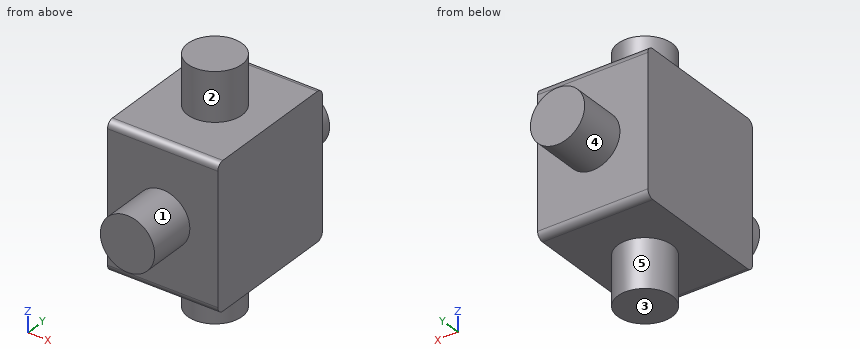
from build123d import *

# Parameters (mm, degrees)
SZKIC1_W                    = 13.2
SZKIC1_H                    = 13.2
DODANIE_WYCI_GNI_CIE1_DEPTH = 10.12
SZKIC2_W                    = 2.49
SZKIC2_H                    = 4.45
SZKIC3_W                    = 2.49
SZKIC3_H                    = 4.45
SZKIC4_W                    = 2.49
SZKIC4_H                    = 4.45
SZKIC5_W                    = 2.49
SZKIC5_H                    = 4.45
ZAOKR_GLENIE1_R             = 0.628571429


with BuildPart() as part:
    # Szkic1 → Dodanie-wyciągnięcie1 (new body)
    with BuildSketch(Plane(origin=(5.06, 0, 0), x_dir=(0, 0, -1), z_dir=(1, 0, 0))):
        Rectangle(SZKIC1_W, SZKIC1_H)
    extrude(amount=-DODANIE_WYCI_GNI_CIE1_DEPTH)

    # Szkic2 → Obrót1 (revolve)
    with BuildSketch(Plane(origin=(0, 0, 0), x_dir=(-1, 0, 0), z_dir=(0, 0, -1))):
        with Locations((-1.245, 8.825)):
            Rectangle(SZKIC2_W, SZKIC2_H)
    revolve(axis=Axis((0, 6.6, 0), (0, 1, 0)))

    # Szkic3 → Obrót2 (revolve)
    with BuildSketch(Plane.XZ):
        with Locations((1.245, -8.825)):
            Rectangle(SZKIC3_W, SZKIC3_H)
    revolve(axis=Axis((0, 0, -6.6), (0, 0, -1)))

    # Szkic4 → Obrót3 (revolve)
    with BuildSketch(Plane(origin=(0, 0, 0), x_dir=(-1, 0, 0), z_dir=(0, 0, -1))):
        with Locations((-1.245, -8.825)):
            Rectangle(SZKIC4_W, SZKIC4_H)
    revolve(axis=Axis((0, -11.05, 0), (0, 1, 0)))

    # Szkic5 → Obrót4 (revolve)
    with BuildSketch(Plane.XZ):
        with Locations((1.245, 8.825)):
            Rectangle(SZKIC5_W, SZKIC5_H)
    revolve(axis=Axis((0, 0, 11.05), (0, 0, -1)))

    # Zaokrąglenie1
    zaokr_glenie1_edges = [part.edges().sort_by_distance(p)[0] for p in [
        (0, 6.6, -6.6),
        (0, -6.6, -6.6),
        (0, -6.6, 6.6),
        (0, 6.6, 6.6),
    ]]
    fillet(zaokr_glenie1_edges, radius=ZAOKR_GLENIE1_R)


solid = part.part
Check sheet for the modelled part. Datum: model origin and axes. Units: mm. Face numbers are marked on the shaded views. A direction names the side the tool comes from. Round coordinates to 2 decimals unless told otherwise and drop trailing zeros. Order: outer loops, then holes, each group sorted by start corner. A loop starts at its lowest first (then second) coordinate and runs counter-clockwise, first axis right, second up. Notation, with made-up numbers: M 44.25,33 L 85.25,33 A21 cw 85.25,48 Z; hole C 29.5,-29.75 d5. An arc over 180 degrees is marked long. One line per item, written item: value. Start each with the question number.
1. Section check A-A on x = 0. Enter the section's corners in (y, z), and give its area (3 significant figures).
2. Gauge pin test, flat ends, axial feed: P1, Ø1, axis at x = -2.5, y = 2.5, coming from the -Z side; P2, Ø2, axis at x = 2, z = -8.5, coming from the +Y side. Record the tip position at first contact, or that the pin passes through.
3. Section check D-D on x = -1.25. Enter the section's corners in (y, z).
4. Section check B-B on z = 0. Enter the section's corners in (x, y), and give its area (3 significant figures).
5. Access from +Z, -Z, +X, -X, +Y, -Y to the whole of each face (thin tool, end or side, straight path). Record for the marked faces 1, 2, 3, 4 and 5.
6. Scan lines: line 1 along Z through (x, y) = (3, 1); line 2 along Z through (x, y) = (-2.25, -7). Record each from-to range of solid material in increasing order.
Results found:
1. outline: M -11.05,-2.49 L -6.6,-2.49 L -6.6,-5.97 A0.63 ccw -5.97,-6.6 L -2.49,-6.6 L -2.49,-11.05 L 2.49,-11.05 L 2.49,-6.6 L 5.97,-6.6 A0.63 ccw 6.6,-5.97 L 6.6,-2.49 L 11.05,-2.49 L 11.05,2.49 L 6.6,2.49 L 6.6,5.97 A0.63 ccw 5.97,6.6 L 2.49,6.6 L 2.49,11.05 L -2.49,11.05 L -2.49,6.6 L -5.97,6.6 A0.63 ccw -6.6,5.97 L -6.6,2.49 L -11.05,2.49 Z
1. area: 263 mm^2
2. P1: z = -6.6
2. P2: y = 2.28
3. outline: M -11.05,-2.15 L -6.6,-2.15 L -6.6,-5.97 A0.63 ccw -5.97,-6.6 L -2.15,-6.6 L -2.15,-11.05 L 2.15,-11.05 L 2.15,-6.6 L 5.97,-6.6 A0.63 ccw 6.6,-5.97 L 6.6,-2.15 L 11.05,-2.15 L 11.05,2.15 L 6.6,2.15 L 6.6,5.97 A0.63 ccw 5.97,6.6 L 2.15,6.6 L 2.15,11.05 L -2.15,11.05 L -2.15,6.6 L -5.97,6.6 A0.63 ccw -6.6,5.97 L -6.6,2.15 L -11.05,2.15 Z
4. outline: M -5.06,-6.6 L -2.49,-6.6 L -2.49,-11.05 L 2.49,-11.05 L 2.49,-6.6 L 5.06,-6.6 L 5.06,6.6 L 2.49,6.6 L 2.49,11.05 L -2.49,11.05 L -2.49,6.6 L -5.06,6.6 Z
4. area: 178 mm^2
5. face 1: -Y
5. face 2: +Z
5. face 3: -Z, +X, -X, +Y, -Y
5. face 4: +Y
5. face 5: -Z
6. line 1: -6.6 to 6.6
6. line 2: -1.07 to 1.07
